Autodesk Fusion 360 part; units mm, degrees
sketch "Sketch1" plane through (0, 0, 0) normal (0, 1, 0) x (1, 0, 0)
  line L0 (0, 0) -> (50, 0)
  line L1 (50, 0) -> (50, -24)
  line L2 (50, -24) -> (0, -24)
  line L3 (0, -24) -> (0, 0)
extrude "Extrude1" add sketch "Sketch1" along normal blind 2
sketch "Sketch2" plane through (0, 0, 0) normal (0, 1, 0) x (1, 0, 0)
  line L0 (0, -24) -> (50, -24)
  line L1 (50, -24) -> (50, -22)
  line L2 (50, -22) -> (0, -22)
  line L3 (0, -22) -> (0, -24)
extrude "Extrude2" add sketch "Sketch2" against normal blind 15
sketch "Sketch3" plane through (0, 0, 0) normal (0, 1, 0) x (1, 0, 0)
  line L0 (17, -20) -> (19, -20)
  line L1 (19, -20) -> (19, -8)
  line L2 (19, -8) -> (17, -8)
  line L3 (17, -8) -> (17, -20)
extrude "Extrude3" cut sketch "Sketch3" along normal blind 5
sketch "Sketch4" plane through (0, 0, 0) normal (0, 1, 0) x (1, 0, 0)
  line L0 (33, -20) -> (31, -20)
  line L1 (31, -20) -> (31, -8)
  line L2 (31, -8) -> (33, -8)
  line L3 (33, -8) -> (33, -20)
extrude "Extrude4" cut sketch "Sketch4" along normal blind 3
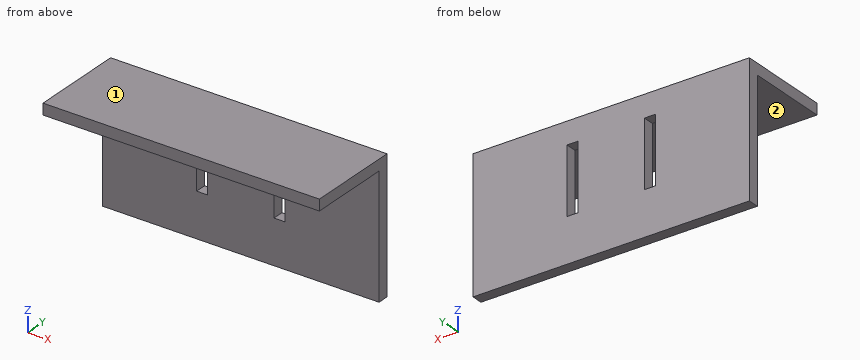
Build history of the part. All positions in model axes, mm. Face numbers are marked on the shaded views. A direction names the side the tool comes from. Round coordinates to 2 decimals unless told otherwise and drop trailing zeros. Loops run counter-clockwise (first coordinate to the right, second up) from the corner with the lowest first, then second, coordinate; pieces in that order, holes last.
Item 1: Drill centre lines: line 1 along Z through (x, y) = (8.5, -13); line 2 along Y through (x, z) = (42.5, 19.5). Where is each one in solid material? Low to high.
Item 2: Saw through at D-D (z = 5). List the corners of the cut face in (x, y), then the cut area to 3 significant figures.
Item 3: Which spindle directions (+Z, -Z, +X, -X, +Y, -Y) get a long thin tool onto all of the face, cutting with end or side? Do the marked faces 1 and 2. Say none if no direction does.
Item 4: Pin check, flat tips, straight feed: P1, Ø1.5, axis at y = -1.5, z = 13, coming from the +X side; P2, Ø5, axis at x = 41, z = 10.5, coming from the -Y side; P3, Ø7.5, axis at x = 27.5, y = -4, coming from the -Z side. Stop position of each tip, or through.
Item 5: Saw through at A-A (z = 11). List the corners of the cut face in (x, y).
Item 6: Saw through at C-C (x = 20.5). List the corners of the cut face in (y, z).
Item 7: Saw through at B-B (y = 0.75). List the corners of the cut face in (x, z), then the cut area to 3 significant figures.
Worked answers:
1. line 1: z = 22 to 24
1. line 2: y = 0 to 2
2. outline: (0, 0) - (50, 0) - (50, 2) - (0, 2) - close
2. area: 100 mm2
3. face 1: +Z, +X, -X, +Y, -Y
3. face 2: -Z, +X, -X, -Y
4. P1: passes through
4. P2: stops at y = 0
4. P3: stops at z = 22
5. outline: (0, 0) - (17, 0) - (17, 2) - (0, 2) - close; (19, 0) - (31, 0) - (31, 2) - (19, 2) - close; (33, 0) - (50, 0) - (50, 2) - (33, 2) - close
6. outline: (-15, 22) - (0, 22) - (0, 0) - (2, 0) - (2, 24) - (-15, 24) - close
7. outline: (0, 0) - (50, 0) - (50, 24) - (0, 24) - close; hole (17, 8) - (19, 8) - (19, 20) - (17, 20) - close; hole (31, 8) - (33, 8) - (33, 20) - (31, 20) - close
7. area: 1,150 mm2
